from build123d import *

# Parameters (mm, degrees)
BOSS_EXTRUDE1_DEPTH = 2.4
BOSS_EXTRUDE2_DEPTH = 4


with BuildPart() as part:
    # Sketch1 → Boss-Extrude1 (new body)
    with BuildSketch(Plane(origin=(0, 0, 0), x_dir=(1, 0, 0), z_dir=(0, 1, 0))):
        Polygon((-27.5, 24.5), (-24.5, 27.5), (24.5, 27.5), (27.5, 24.5), (27.5, -24.5), (24.5, -27.5), (-24.5, -27.5), (-27.5, -24.5), align=None)
    extrude(amount=BOSS_EXTRUDE1_DEPTH)

    # Sketch2 → Boss-Extrude2 (add)
    with BuildSketch(Plane(origin=(0, 2.4, 0), x_dir=(1, 0, 0), z_dir=(0, 1, 0))):
        with BuildLine():
            Line((-24, -20.465570271), (-24, 20.465570271))
            ThreePointArc((-24, 20.465570271), (-25, 21.465570271), (-26, 20.465570271))
            Line((-26, 20.465570271), (-26, -20.465570271))
            ThreePointArc((-26, -20.465570271), (-25, -21.465570271), (-24, -20.465570271))
        make_face()
        with BuildLine():
            Line((-20.465570271, 24), (20.465570271, 24))
            ThreePointArc((20.465570271, 24), (21.465570271, 25), (20.465570271, 26))
            Line((20.465570271, 26), (-20.465570271, 26))
            ThreePointArc((-20.465570271, 26), (-21.465570271, 25), (-20.465570271, 24))
        make_face()
        with BuildLine():
            Line((24, 20.465570271), (24, -20.465570271))
            ThreePointArc((24, -20.465570271), (25, -21.465570271), (26, -20.465570271))
            Line((26, -20.465570271), (26, 20.465570271))
            ThreePointArc((26, 20.465570271), (25, 21.465570271), (24, 20.465570271))
        make_face()
        with BuildLine():
            Line((20.465570271, -24), (-20.465570271, -24))
            ThreePointArc((-20.465570271, -24), (-21.465570271, -25), (-20.465570271, -26))
            Line((-20.465570271, -26), (20.465570271, -26))
            ThreePointArc((20.465570271, -26), (21.465570271, -25), (20.465570271, -24))
        make_face()
    extrude(amount=BOSS_EXTRUDE2_DEPTH)


solid = part.part
Can you work these out from the model? Positions are in its coordinate system, mm. A direction names the side the tool comes from. Round coordinates to 2 decimals unless told otherwise and drop trailing zeros. Write each loop counter-clockwise with the first axis right and the second up, starting at its lowest first coordinate (ties: lowest second). Pieces come first, ordered by that corner, then holes. Notation, with made-up numbers: M -27.75,-7.75 L -19.75,-7.75 A11 ccw -19.75,13.25 Z; hole C 6.25,57 d9. An arc over 180 degrees is marked long. Use CSV: the item, a comma, the result in double quotes.
(1) We'd pull the mould along Z, two halves only. Please class faces 6 (the cylindrical face through (25.022, 4.372, -21.465)), 7 (the flat face through (24, 4, 0)), 8 (the flat face through (0, 2.4, 0)): +Z half, -Z half, draft (parallel to the pull), parting line (faces both ways), or undercut.
Check values:
face 6,"-Z half"
face 7,"draft"
face 8,"undercut"
(2) Imagine slicing it at B-B (x = -8). Write out the boundary of the cut face in (y, z), plus the area to 3 significant figures.
Check values:
outline,"M 0,-27.5 L 2.4,-27.5 L 2.4,-26 L 6.4,-26 L 6.4,-24 L 2.4,-24 L 2.4,24 L 6.4,24 L 6.4,26 L 2.4,26 L 2.4,27.5 L 0,27.5 Z"
area,"148 mm^2"
(3) Imagine slicing it at A-A (y = 5.25). Write out the boundary of the cut face in (x, z), plus the area to 3 significant figures.
Check values:
outline,"M -26,-20.47 A1 ccw -24,-20.47 L -24,20.47 A1 ccw -26,20.47 Z; M -20.47,-26 L 20.47,-26 A1 ccw 20.47,-24 L -20.47,-24 A1 ccw Z; M -20.47,24 L 20.47,24 A1 ccw 20.47,26 L -20.47,26 A1 ccw Z; M 24,-20.47 A1 ccw 26,-20.47 L 26,20.47 A1 ccw 24,20.47 Z"
area,"340 mm^2"
(4) On a 3-axis mill with a long thin cutter (end or side, diameter ignored), from which of +Z, -Z, +X, -X, +Y, -Y can I reach the whole of each face in a straight line? I mean faces 1 (the flat face through (0, 4, 26)), 2 (the flat face through (-24, 4, 0)), 3 (the cylindrical face through (24.978, 4.372, 21.465)), 4 (the cylindrical face through (21.465, 4.372, 25.022)), 5 (the flat face through (0, 4, -26)). Say none if no direction works.
Check values:
face 1,"+Z, +X, -X, +Y"
face 2,"+Z, -Z, +Y"
face 3,"+Z, +Y"
face 4,"+X, +Y"
face 5,"-Z, +X, -X, +Y"
(5) I'm going to push flat-ended pins straight in: pin 1 (1.5 mm diameter, centred on x = -10, y = 2.5, fed in from -Z); pin 2 (2 mm diameter, centred on x = -5.5, y = 3.5, fed in from -Z); pin 3 (2 mm diameter, centred on y = 4.5, z = 0.5, fed in from +X); pin 4 (1.5 mm diameter, centred on x = -0.5, z = -2.5, fed in from +Y). Where does each tip first touch, or does it pass through?
Check values:
pin 1,"z = -27.5"
pin 2,"z = -26"
pin 3,"x = 26"
pin 4,"y = 2.4"
(6) I need wall thicknesses on line 1 along Z through (x, y) = (16.5, 6.25); line 2 along Y through (x, z) = (-14, 8.5). Which ranges of each line are inside material? Lowest first, please.
Check values:
line 1,"-26 to -24, 24 to 26"
line 2,"0 to 2.4"
